Design review of the part shown in the three views and the two pictorial views. Dimensions are in mm from the part's minimum x, y and z. A direction names the side the tool comes from. Give positions to 0.01 mm unless a question says otherwise; leave off trailing zeros. Write each loop counter-clockwise with the first axis right and the second up, starting at its lowest first coordinate (ties: lowest second). Pieces come first, ordered by that corner, then holes.
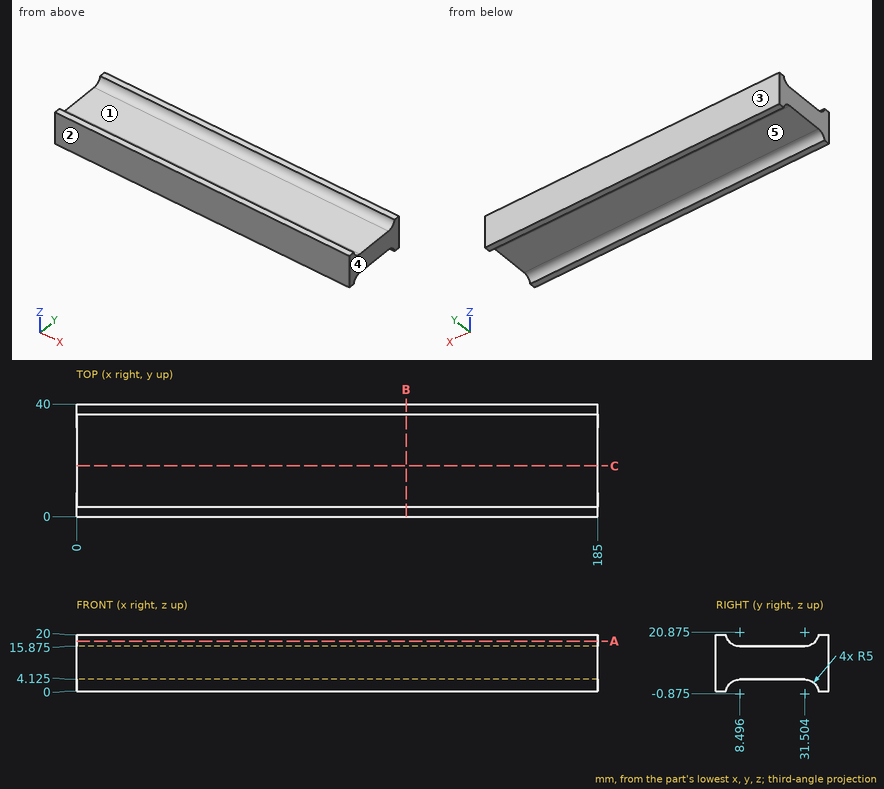
(1) To check wall thickness, follow L1, parallel to Z at x = 51, y = 15 (3 decimals); L2, parallel to Y at x = 67, z = 18.5; L3, parallel to Y at x = 47, z = 18.75. State the ranges of each line that lie inside material, in increasing order.
Resolved:
L1: z = 4.125 to 15.875
L2: y = 0 to 4.1, 35.9 to 40
L3: y = 0 to 3.97, 36.03 to 40
(2) Clearance check with flat-ended pins moving along their axes: P1, Ø18.5, axis at x = 63, y = 18, coming from the -Z side (3 decimals); P2, Ø6, axis at x = 38, y = 26, coming from the +Z side (3 decimals). State where each tip first meets the part, or that it passes through.
Resolved:
P1: stops at z = 4.125
P2: stops at z = 15.875
(3) Mouldability with a two-part tool opening along Y and no side actions: class the marked faces 3, 4 and 5 as pulls with the +Y half, pulls with the -Y half, needs draft (parallel to the pull), parting line crosses it, or undercut.
Resolved:
face 3: pulls with the +Y half
face 4: needs draft
face 5: undercut
(4) Consider section B-B, the plane x = 117. Give the boundary of the cut face in (y, z) (1 decimal).
Resolved:
outline: (0, 0) - (3.6, 0) arc R5 cw to (8.5, 4.1) - (31.5, 4.1) arc R5 cw to (36.4, 0) - (40, 0) - (40, 20) - (36.4, 20) arc R5 cw to (31.5, 15.9) - (8.5, 15.9) arc R5 cw to (3.6, 20) - (0, 20) - close
(5) Consider section C-C, the plane y = 18. Give the boundary of the cut face in (x, z) (3 decimals), then the cut area to 3 significant figures.
Resolved:
outline: (0, 4.125) - (185, 4.125) - (185, 15.875) - (0, 15.875) - close
area: 2,170 mm2
(6) Consider section A-A, the plane z = 17.75. Give the boundary of the cut face in (x, y).
Resolved:
outline: (0, 0) - (185, 0) - (185, 4.59) - (0, 4.59) - close; (0, 35.41) - (185, 35.41) - (185, 40) - (0, 40) - close
(7) Tool access review of the marked faces 1 and 2: name each direction out of +Z, -Z, +X, -X, +Y, -Y from which nothing blocks a thin tool from reaching the whole face with its end or side.
Resolved:
face 1: +Z, +X, -X
face 2: +Z, -Z, +X, -X, -Y
